The model under review builds one solid part; all positions refer to its coordinate system, in mm. A direction names the side the tool comes from. Coordinates: 2 decimals unless noted, no trailing zeros. Write each loop counter-clockwise with the first axis right and the second up, starting at its lowest first coordinate (ties: lowest second). Pieces come first, ordered by that corner, then holes. Notation, with made-up numbers: (52.5, 82.25) - (104.5, 82.25) arc R26 cw to (104.5, 112.25) - close; hole circle Ø8 at (84.5, 55.25). An arc over 180 degrees is marked (long way). Put each result on its own line as item: value.
from build123d import *

# Parameters (mm, degrees)
SKETCH2_R               = 97.5
SKETCH2_R_2             = 92.5
BOSS_EXTRUDE1_DEPTH     = 70
SKETCH3_W               = 110
SKETCH3_H               = 114
CUT_EXTRUDE1_DEPTH      = 98.5
SKETCH4_W               = 100
SKETCH4_H               = 120
CUT_EXTRUDE2_DEPTH      = 98.5
CUT_EXTRUDE2_DEPTH_BACK = 98.5
SKETCH5_W               = 61
SKETCH5_H               = 20.506210941
CUT_EXTRUDE3_DEPTH      = 98.5
CUT_EXTRUDE3_DEPTH_BACK = 98.5
SKETCH6_R               = 9.784293737
CUT_EXTRUDE4_DEPTH      = 98.5
BOSS_EXTRUDE2_DEPTH     = 70
SKETCH9_R               = 2
CUT_EXTRUDE5_DEPTH      = 71.0000001


with BuildPart() as part:
    # Sketch2 → Boss-Extrude1 (new body)
    with BuildSketch(Plane.XY):
        Circle(SKETCH2_R)
        Circle(SKETCH2_R_2, mode=Mode.SUBTRACT)
    extrude(amount=BOSS_EXTRUDE1_DEPTH)

    # Sketch3 → Cut-Extrude1 (cut, through all)
    with BuildSketch(Plane(origin=(0, 0, 0), x_dir=(1, 0, 0), z_dir=(0, 1, 0))):
        with Locations((0, -70)):
            Rectangle(SKETCH3_W, SKETCH3_H)
    extrude(amount=-CUT_EXTRUDE1_DEPTH, mode=Mode.SUBTRACT)

    # Sketch4 → Cut-Extrude2 (cut, two sides)
    with BuildSketch(Plane(origin=(0, 0, 0), x_dir=(0, 0, -1), z_dir=(1, 0, 0))) as cut_extrude2_sk:
        with Locations((-70, 0)):
            Rectangle(SKETCH4_W, SKETCH4_H)
    extrude(amount=CUT_EXTRUDE2_DEPTH, mode=Mode.SUBTRACT)
    extrude(cut_extrude2_sk.sketch, amount=-CUT_EXTRUDE2_DEPTH_BACK, mode=Mode.SUBTRACT)

    # Sketch5 → Cut-Extrude3 (cut, two sides)
    with BuildSketch(Plane(origin=(0, 0, 0), x_dir=(0, 0, -1), z_dir=(1, 0, 0))) as cut_extrude3_sk:
        with Locations((-39.5, -70.253105471)):
            Rectangle(SKETCH5_W, SKETCH5_H)
    extrude(amount=CUT_EXTRUDE3_DEPTH, mode=Mode.SUBTRACT)
    extrude(cut_extrude3_sk.sketch, amount=-CUT_EXTRUDE3_DEPTH_BACK, mode=Mode.SUBTRACT)

    # Sketch6 → Cut-Extrude4 (cut, through all)
    with BuildSketch(Plane(origin=(0, 0, 0), x_dir=(1, 0, 0), z_dir=(0, 1, 0))):
        with Locations((0, -56.012862066)):
            Circle(SKETCH6_R)
    extrude(amount=CUT_EXTRUDE4_DEPTH, mode=Mode.SUBTRACT)

    # Sketch8 → Boss-Extrude2 (add)
    with BuildSketch(Plane.XY):
        with BuildLine():
            ThreePointArc((66.0209996, 64.787943414), (54.682390857, 64.138601978), (53.530180965, 75.437190602))
            ThreePointArc((53.530180965, 75.437190602), (60.012272162, 70.390178221), (66.0209996, 64.787943414))
        make_face()
    boss_extrude2 = extrude(amount=BOSS_EXTRUDE2_DEPTH)

    # Sketch9 → Cut-Extrude5 (cut, through all)
    with BuildSketch(Plane(origin=(0, 0, 0), x_dir=(-1, 0, 0), z_dir=(0, 0, -1))):
        with Locations((-59.32689754, 69.571871503)):
            Circle(SKETCH9_R)
    cut_extrude5 = extrude(amount=-CUT_EXTRUDE5_DEPTH, mode=Mode.SUBTRACT)

    # Mirror1: Boss-Extrude2, Cut-Extrude5 across plane
    add(boss_extrude2.mirror(Plane(origin=(0, 0, 0), x_dir=(0, 0, 1), z_dir=(1, 0, 0))))
    add(cut_extrude5.mirror(Plane(origin=(0, 0, 0), x_dir=(0, 0, 1), z_dir=(1, 0, 0))), mode=Mode.SUBTRACT)


solid = part.part
1. Consider section A-A on x = 0. State the section outline as (y, z) points, plus the area to 3 significant figures.
Determined:
outline: (-97.5, 0) - (-92.5, 0) - (-92.5, 13) - (-97.5, 13) - close; (92.5, 0) - (97.5, 0) - (97.5, 46.23) - (92.5, 46.23) - close; (92.5, 65.8) - (97.5, 65.8) - (97.5, 70) - (92.5, 70) - close
area: 317 mm^2
2. Machinability: for faces 5 (the flat face through (-63, -71, 9)), 6 (the cylindrical face through (0.799, 92.497, 34.51)), 7 (the flat face through (-74, -60, 15)), which of the approach directions +Z, -Z, +X, -X, +Y, -Y give a long, thin tool a straight path to every point of the face, cutting with its end or side? Answer none if there is none.
Determined:
face 5: +Z, +X, -X
face 6: +Z, -Z
face 7: +Z, +X, -X, -Y
3. Consider section C-C on x = 34. State the section outline as (y, z) points.
Determined:
outline: (-91.38, 0) - (-86.02, 0) - (-86.02, 13) - (-91.38, 13) - close; (86.02, 0) - (91.38, 0) - (91.38, 70) - (86.02, 70) - close
4. To check wall thickness, follow probe 1 along Z at (x, y) = (0, 94.9); probe 2 along X at (y, z) = (0.5, 5); probe 3 along Y at (x, z) = (0, 30). State the ranges of each line that lie inside material, in increasing order.
Determined:
probe 1: z = 0 to 46.23, 65.8 to 70
probe 2: x = -97.5 to -92.5, 92.5 to 97.5
probe 3: y = 92.5 to 97.5
5. Consider section B-B on y = 0. State the section outline as (x, z) points, plus the area to 3 significant figures.
Determined:
outline: (-97.5, 0) - (-92.5, 0) - (-92.5, 20) - (-97.5, 20) - close; (92.5, 0) - (97.5, 0) - (97.5, 20) - (92.5, 20) - close
area: 200 mm^2
6. For pin 1 Ø7 at (x, z) = (73, 33) entering from -Y; pin 2 Ø12 at (x, z) = (-42.5, 37) entering from +Y; pin 3 Ø22.5 at (x, y) = (68, -72) entering from +Z, all flat-tipped, find the tip position at first contact; note any pin that passes through.
Determined:
pin 1: stops at y = 60
pin 2: stops at y = 90.41
pin 3: stops at z = 9
7. Consider section D-D on z = 63. State the section outline as (x, y) points, plus the area to 3 significant figures.
Determined:
outline: (-76.85, 60) - (-70.4, 60) arc R92.5 cw to (-66.02, 64.79) arc R8.22 ccw to (-53.53, 75.44) arc R92.5 cw to (-6.85, 92.25) - (-6.85, 97.26) arc R97.5 ccw to start; (6.85, 92.25) arc R92.5 cw to (53.53, 75.44) arc R8.22 ccw to (66.02, 64.79) arc R92.5 cw to (70.4, 60) - (76.85, 60) arc R97.5 ccw to (6.85, 97.26) - close; hole circle Ø4 at (-59.33, 69.57); hole circle Ø4 at (59.33, 69.57)
area: 957 mm^2
8. The part is to be moulded in two halves that separate along Y. For faces 1 (the flat face through (63, -71, 9)), 2 (the flat face through (74, -60, 15)), 3 (the cylindrical face through (-16.996, -90.925, 11.503)), 4 (the cylindrical face through (-9.775, 94.702, 55.583)), say which applies: +Y half, -Y half, draft (parallel to the pull), parting line (faces both ways), or undercut.
Determined:
face 1: undercut
face 2: -Y half
face 3: undercut
face 4: draft
